from build123d import *

# Parameters (mm, degrees)
ESQUISSE1_R             = 4
BOSS_EXTRU_1_DEPTH      = 40
ESQUISSE3_R             = 2
ENL_V_MAT_EXTRU_1_DEPTH = 10
ESQUISSE4_R             = 2
BOSS_EXTRU_2_DEPTH      = 5


with BuildPart() as part:
    # Esquisse1 → Boss.-Extru.1 (new body)
    with BuildSketch(Plane(origin=(0, 0, 0), x_dir=(1, 0, 0), z_dir=(0, 1, 0))):
        Circle(ESQUISSE1_R)
    extrude(amount=-BOSS_EXTRU_1_DEPTH)

    # Esquisse3 → Enlèv. mat.-Extru.1 (cut)
    with BuildSketch(Plane(origin=(0, 0, 0), x_dir=(1, 0, 0), z_dir=(0, 1, 0))):
        Circle(ESQUISSE3_R)
    extrude(amount=-ENL_V_MAT_EXTRU_1_DEPTH, mode=Mode.SUBTRACT)

    # Esquisse4 → Boss.-Extru.2 (add)
    with BuildSketch(Plane.XZ.offset(40)):
        Circle(ESQUISSE4_R)
    extrude(amount=BOSS_EXTRU_2_DEPTH)


solid = part.part
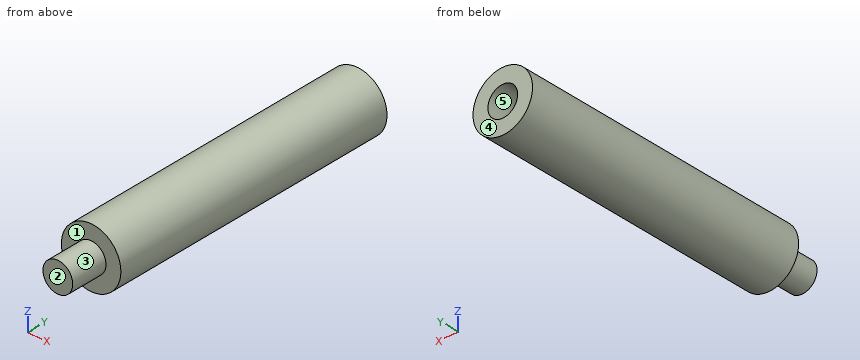
Source: CAD feature listing. Evaluate the final solid. Frame: model axes, mm. Face numbers are marked on the shaded views. A direction names the side the tool comes from. Give positions to 0.01 mm unless a question says otherwise; leave off trailing zeros. Write each loop counter-clockwise with the first axis right and the second up, starting at its lowest first coordinate (ties: lowest second). Pieces come first, ordered by that corner, then holes. Notation, with made-up numbers: M 75.25,26.5 L 80.25,26.5 A13 ccw 80.25,40.5 Z; hole C -23.5,62 d10. An arc over 180 degrees is marked long. Return JSON: item names as keys, results as strings. Group by question number.
1) Cut plane D-D, the plane y = -33.5. Output: boundary loops of the cut face in (x, z), then the cut area to 3 significant figures.
2) Cut plane A-A, the plane x = 0. Output: boundary loops of the cut face in (y, z), then the cut area to 3 significant figures.
3) Ray query, L1, parallel to X at y = -2.25, z = 0; L2, parallel to Y at x = -1.5, z = 2.25. Return the intervals inside material, ascending.
4) Cut plane C-C, the plane y = -6.5. Output: boundary loops of the cut face in (x, z).
5) Cut plane B-B, the plane z = 0. Output: boundary loops of the cut face in (x, y).
6) First-contact query: pin 1 Ø1.5 at (y, z) = (-14, -2.5) entering from -X; pin 2 Ø1 at (x, y) = (-3, -31.5) entering from -Z; pin 3 Ø1.2 at (x, z) = (0, 0) entering from +Y. Flat tips, straight axial feed; report the tip coordinate or a pass-through.
7) Set-up query: the marked faces 1 and 2. Return all of +Z, -Z, +X, -X, +Y, -Y with unobstructed straight access to the full face (end or side cutting, diameter ignored); none if empty.
8) Draft query along Z for the marked faces 3, 4 and 5. Return one class per face: released by +Z, released by -Z, zero draft, split by the parting line, or undercut.
Data:
{
 "1": {"outline": "C 0,0 d8", "area": "50.3 mm²"},
 "2": {"outline": "M -45,-2 L -40,-2 L -40,-4 L 0,-4 L 0,-2 L -10,-2 L -10,2 L 0,2 L 0,4 L -40,4 L -40,2 L -45,2 Z", "area": "300 mm²"},
 "3": {"L1": "x = -4 to -2, 2 to 4", "L2": "y = -40 to 0"},
 "4": {"outline": "C 0,0 d8; hole C 0,0 d4"},
 "5": {"outline": "M -4,-40 L -2,-40 L -2,-45 L 2,-45 L 2,-40 L 4,-40 L 4,0 L 2,0 L 2,-10 L -2,-10 L -2,0 L -4,0 Z"},
 "6": {"pin 1": "stops at x = -3.6", "pin 2": "stops at z = -3.12", "pin 3": "stops at y = -10"},
 "7": {"face 1": "-Y", "face 2": "+Z, -Z, +X, -X, -Y"},
 "8": {"face 3": "split by the parting line", "face 4": "zero draft", "face 5": "undercut"}
}
